```python
from build123d import *

# Parameters (mm, degrees)
F0_W     = 863.6
F0_H     = 508
F1_DEPTH = 19.05
F2_W     = 19.05
F2_H     = 361.95
F3_DEPTH = 12.7
F4_R     = 57.15
F5_DEPTH = 25.4


with BuildPart() as f1:
    # F0 (on Top) → F1 (new body)
    with BuildSketch(Plane.XY):
        Rectangle(F0_W, F0_H)
    extrude(amount=F1_DEPTH)

    # F2 (on face) → F3 (cut)
    with BuildSketch(Plane(origin=(0, 0, 0), x_dir=(1, 0, 0), z_dir=(0, 0, -1))):
        Polygon((-304.8, -209.55), (381, -209.55), (381, -190.5), (361.95, -190.5), (139.7, -190.5), (120.65, -190.5), (-285.75, -190.5), (-304.8, -190.5), align=None)
        with Locations((371.475, -9.525)):
            Rectangle(F2_W, F2_H)
        with Locations((-295.275, -9.525)):
            Rectangle(F2_W, F2_H)
        with Locations((130.175, -9.525)):
            Rectangle(F2_W, F2_H)
    extrude(amount=-F3_DEPTH, mode=Mode.SUBTRACT)

    # F4 (on face) → F5 (cut)
    with BuildSketch(Plane.XY.offset(19.05)):
        with Locations((-362.7038, 168.77979)):
            Circle(F4_R)
    extrude(amount=-F5_DEPTH, mode=Mode.SUBTRACT)


solid = f1.part
```
For this review, take the finished solid that the model builds, in its own axes (mm). Round coordinates to 2 decimals unless told otherwise and drop trailing zeros. Write each loop counter-clockwise with the first axis right and the second up, starting at its lowest first coordinate (ties: lowest second). Pieces come first, ordered by that corner, then holes.
1) Take a section at A-A on y = -52. Give the boundary of the cut face in (x, z), then the cut area to 3 significant figures.
Answer below:
outline: (-431.8, 0) - (-304.8, 0) - (-304.8, 12.7) - (-285.75, 12.7) - (-285.75, 0) - (120.65, 0) - (120.65, 12.7) - (139.7, 12.7) - (139.7, 0) - (361.95, 0) - (361.95, 12.7) - (381, 12.7) - (381, 0) - (431.8, 0) - (431.8, 19.05) - (-431.8, 19.05) - close
area: 15,700 mm2
2) Take a section at C-C on z = 8.75. Give the boundary of the cut face in (x, y).
Answer below:
outline: (-431.8, -254) - (431.8, -254) - (431.8, 254) - (-431.8, 254) - close; hole circle Ø114.3 at (-362.7, 168.78); hole (-304.8, -171.45) - (-285.75, -171.45) - (-285.75, 190.5) - (120.65, 190.5) - (120.65, -171.45) - (139.7, -171.45) - (139.7, 190.5) - (361.95, 190.5) - (361.95, -171.45) - (381, -171.45) - (381, 209.55) - (-304.8, 209.55) - close
3) Take a section at D-D on x = -338. Give the boundary of the cut face in (y, z), then the cut area to 3 significant figures.
Answer below:
outline: (-254, 0) - (117.24, 0) - (117.24, 19.05) - (-254, 19.05) - close; (220.31, 0) - (254, 0) - (254, 19.05) - (220.31, 19.05) - close
area: 7,710 mm2
4) Mouldability with a two-part tool opening along X and no side actions: class faces 1 (the face through (-6, 4, 19.05)), 2 (the face through (431.8, -4, 9)), 3 (the face through (-419.8, 171.3, 9.7)), 4 (the face through (-431.8, -4, 9)) as +X half, -X half, draft (parallel to the pull), parting line (faces both ways), or undercut.
Answer below:
face 1: draft
face 2: +X half
face 3: undercut
face 4: -X half
5) Insertion check: pin 1 Ø8 at (x, y) = (333, 151.5) entering from -Z. The pin has a flat end and moves straight along its axis. Give the tip position at first contact, or say it passes through.
Answer below:
pin 1: stops at z = 0
6) For line 1 along X through (y, z) = (-157.5, 5); line 2 along Y through (x, z) = (107.5, 3.75); line 3 along Y through (x, z) = (373, 3), list the stretches that pass through material, from the lowest coordinate up.
Answer below:
line 1: x = -431.8 to -304.8, -285.75 to 120.65, 139.7 to 361.95, 381 to 431.8
line 2: y = -254 to 190.5, 209.55 to 254
line 3: y = -254 to -171.45, 209.55 to 254
7) Take a section at B-B on x = -249.5. Give the boundary of the cut face in (y, z).
Answer below:
outline: (-254, 0) - (190.5, 0) - (190.5, 12.7) - (209.55, 12.7) - (209.55, 0) - (254, 0) - (254, 19.05) - (-254, 19.05) - close
